Could you check a few things on this model? Use its own coordinates, in mm. Face numbers are marked on the shaded views. A direction names the side the tool comes from. Coordinates: 2 decimals unless noted, no trailing zeros. Write each loop counter-clockwise with the first axis right and the second up, starting at its lowest first coordinate (ties: lowest second). Pieces come first, ordered by that corner, then holes. Notation, with made-up numbers: M -36.75,-17.75 L 11.25,-17.75 A24 cw 11.25,2.25 Z; hole C -17.5,56.25 d8. An arc over 180 degrees is marked long. Write item = value, one per line.
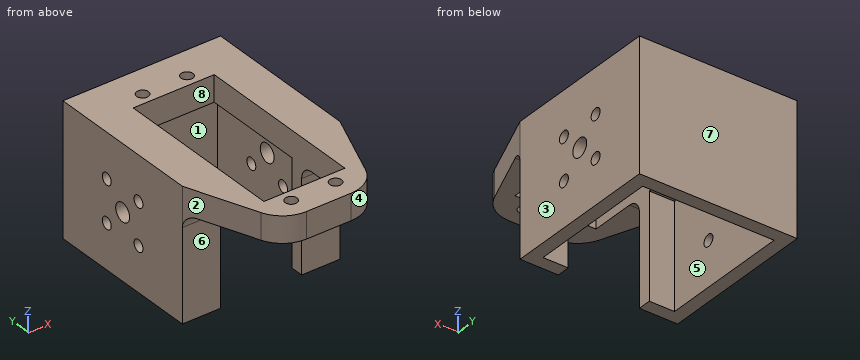
Autodesk Inventor part; units mm, degrees
ref_plane "YZ Plane" through (0, 0, 0) normal (1, 0, 0) x (0, 1, 0)
ref_plane "XZ Plane" through (0, 0, 0) normal (0, 1, 0) x (-1, 0, 0)
ref_plane "XY Plane" through (0, 0, 0) normal (0, 0, 1) x (1, 0, 0)
sketch "Sketch1" plane through (0, 0, 0) normal (0, 0, 1) x (1, 0, 0)
  line L0 (-25.15, 25.15) -> (25.15, 25.15)
  line L1 (25.15, 25.15) -> (25.15, -25.15)
  line L2 (25.15, -25.15) -> (-25.15, -25.15)
  line L3 (-25.15, -25.15) -> (-25.15, 25.15)
  line L4 (-25.15, 25.15) -> (25.15, -25.15) construction
  line L5 (25.15, 25.15) -> (-25.15, -25.15) construction
  line L6 (-30.15, 30.15) -> (30.15, 30.15)
  line L7 (30.15, 30.15) -> (30.15, -30.15)
  line L8 (30.15, -30.15) -> (-30.15, -30.15)
  line L9 (-30.15, -30.15) -> (-30.15, 30.15)
  line L10 (-30.15, 30.15) -> (30.15, -30.15) construction
  line L11 (30.15, 30.15) -> (-30.15, -30.15) construction
  line L12 (0, 25.15) -> (0, 18.5) construction
  line L13 (0, 18.5) -> (8.5, 18.5) construction
  circle A0 centre (8.5, 18.5) radius 2.25
  line L14 (8.5, 18.5) -> (-8.5, 18.5)
  line L15 (-8.5, 18.5) -> (-8.5, -56.5)
  line L16 (-8.5, -56.5) -> (8.5, -56.5)
  line L17 (8.5, -56.5) -> (8.5, 18.5)
  circle A1 centre (8.5, -56.5) radius 2.25
  line L18 (-8.5, 18.5) -> (8.5, -56.5) construction
  line L19 (-15.5, 14) -> (15.5, 14)
  line L20 (15.5, 14) -> (15.5, -52)
  line L21 (15.5, -52) -> (-15.5, -52)
  line L22 (-15.5, -52) -> (-15.5, 14)
  line L23 (-15.5, 14) -> (15.5, -52) construction
  line L24 (15.5, 14) -> (-15.5, -52) construction
  circle A2 centre (-8.5, -56.5) radius 2.25
  circle A3 centre (-8.5, 18.5) radius 2.25
  line L25 (-30.15, -30.15) -> (-20.0032, -56.4398)
  arc A4 (-20.0032, -56.4398) -> (-8.5, -64.3302) centre (-8.5, -52) ccw
  line L26 (0, 0) -> (0, -19) construction
  line L27 (30.15, -30.15) -> (20.0032, -56.4398)
  line L28 (-8.5, -64.3302) -> (8.5, -64.3302)
  arc A5 (8.5, -64.3302) -> (20.0032, -56.4398) centre (8.5, -52) ccw
  point P0 (15.5, -25.15)
  point P1 (15.5, -30.15)
  point P2 (-15.5, -30.15)
  point P3 (-15.5, -25.15)
  dimension "d0" = 50.3
  dimension "d2" = 60.3
  dimension "d4" = 6.65
  dimension "d5" = 8.5
  dimension "d6" = 4.5
  dimension "d7" = 17
  dimension "d8" = 75
  dimension "d10" = 31
  dimension "d11" = 66
extrude "Extrusion1" add sketch "Sketch1" against normal blind 40 contours L3 L2 L22 L8 L9 L6 L7 L20 L1 L0
extrude "Extrusion2" add sketch "Sketch1" along normal blind 10 contours L3 L2 L22 L8 L9 L6 L7 L20 L1 L0 | L0 L1 L2 L20 L19 L17 A0 L14 A3 L15 L22 L3 | L22 L21 L15 A2 L16 A1 L17 L20 L8 L27 A5 L28 A4 L25 | L15 A3 L14 A0 L17 L19 | L21 L17 A1 L16 A2 L15
fillet "Fillet1" radius 5 2 edges at (22.825, -30.15, 0) (-22.825, -30.15, 0)
sketch "Sketch2" plane through (30.15, -30.15, -40) normal (1, 0, 0) x (0, 0, -1)
  line L0 (0, 60.3) -> (0, 0)
  line L1 (-10, 60.3) -> (-40, 60.3)
  line L2 (-40, 60.3) -> (-40, 0)
  line L3 (-40, 0) -> (-10, 0)
  line L4 (-10, 0) -> (-10, 60.3)
  line L5 (-35, 0) -> (0, 0) construction
  circle A0 centre (-25, 30.15) radius 3.5
  line L6 (0.0184, 0) -> (-9.9816, 0) construction
  line L7 (-35, 0) -> (0, 0)
  line L8 (-33, 38.15) -> (-17, 38.15) construction
  line L9 (-17, 38.15) -> (-17, 22.15) construction
  line L10 (-17, 22.15) -> (-33, 22.15) construction
  line L11 (-33, 22.15) -> (-33, 38.15) construction
  line L12 (-33, 38.15) -> (-17, 22.15) construction
  line L13 (-17, 38.15) -> (-33, 22.15) construction
  circle A1 centre (-33, 38.15) radius 2.25
  circle A2 centre (-17, 38.15) radius 2.25
  circle A3 centre (-17, 22.15) radius 2.25
  circle A4 centre (-33, 22.15) radius 2.25
  line L14 (-25, 30.15) -> (-20.3356, 34.8144) construction
  line L15 (-10, 60.3) -> (-40, 0) construction
  line L16 (-25, 30.15) -> (-30.0486, 30.15) construction
  point P0 (-40, 30.15)
  dimension "d20" = 30
  dimension "d21" = 7
  dimension "d24" = 10
  dimension "d25" = 16
  dimension "d27" = 4.5
  dimension "d28" = 60.3
extrude "Extrusion3" cut sketch "Sketch2" against normal blind 65 contours A0 | A1 | A2 | A3 | A4
properties part number "Servo-house" material "PBT Plastic"
Item 1: Imagine slicing it at A-A (y = 8). Write out the boundary of the cut face in (x, z).
Numbers:
outline = M -30.15,-40 L -25.15,-40 L -25.15,-25.25 L -30.15,-25.25 Z; M -30.15,-20.75 L -25.15,-20.75 L -25.15,-9.25 L -30.15,-9.25 Z; M -30.15,-4.75 L -25.15,-4.75 L -25.15,0 L -15.5,0 L -15.5,10 L -30.15,10 Z; M 15.5,0 L 25.15,0 L 25.15,-4.75 L 30.15,-4.75 L 30.15,10 L 15.5,10 Z; M 25.15,-40 L 30.15,-40 L 30.15,-25.25 L 25.15,-25.25 Z; M 25.15,-20.75 L 30.15,-20.75 L 30.15,-9.25 L 25.15,-9.25 Z
Item 2: I'm going to push flat-ended pins straight in: P1, Ø6, axis at y = 8, z = -7, coming from the +X side; P2, Ø1, axis at x = 21, y = -4.5, coming from the -Z side; P3, Ø11.5, axis at x = 20.5, z = -21, coming from the -Y side. Where does each tip first touch, or does it pass through?
Numbers:
P1 = 30.15
P2 = 0
P3 = -30.15
Item 3: Imagine slicing it at C-C (z = -23). Write out the boundary of the cut face in (x, y), and give its area (3 significant figures).
Numbers:
outline = M -30.15,-30.15 L -15.5,-30.15 L -15.5,-25.15 L -25.15,-25.15 L -25.15,-10.25 L -30.15,-10.25 Z; M -30.15,-5.75 L -25.15,-5.75 L -25.15,5.75 L -30.15,5.75 Z; M -30.15,10.25 L -25.15,10.25 L -25.15,25.15 L 25.15,25.15 L 25.15,10.25 L 30.15,10.25 L 30.15,30.15 L -30.15,30.15 Z; M 15.5,-30.15 L 30.15,-30.15 L 30.15,-10.25 L 25.15,-10.25 L 25.15,-25.15 L 15.5,-25.15 Z; M 25.15,-5.75 L 30.15,-5.75 L 30.15,5.75 L 25.15,5.75 Z
area = 861 mm²
Item 4: Imagine slicing it at D-D (y = 18.5). Write out the boundary of the cut face in (x, z), and give its area (3 significant figures).
Numbers:
outline = M -30.15,-40 L -25.15,-40 L -25.15,0 L -10.75,0 L -10.75,10 L -30.15,10 Z; M -6.25,0 L 6.25,0 L 6.25,10 L -6.25,10 Z; M 10.75,0 L 25.15,0 L 25.15,-40 L 30.15,-40 L 30.15,10 L 10.75,10 Z
area = 913 mm²
Item 5: If I drill on line 1 along Y through (x, z) = (26, -23); line 2 along Y through (x, z) = (-18, -29); line 3 along Y through (x, z) = (-8.5, 4), over which ranges is the centre line in solid material (lowest first)?
Numbers:
line_1 = -30.15 to -10.25, -5.75 to 5.75, 10.25 to 30.15
line_2 = -30.15 to -25.15, 25.15 to 30.15
line_3 = -64.33 to -58.75, -54.25 to -52, 14 to 16.25, 20.75 to 30.15
Item 6: Imagine slicing it at B-B (x = -2.5). Write out the boundary of the cut face in (y, z), and give its area (3 significant figures).
Numbers:
outline = M -64.33,0 L -52,0 L -52,10 L -64.33,10 Z; M 14,0 L 25.15,0 L 25.15,-40 L 30.15,-40 L 30.15,10 L 14,10 Z
area = 485 mm²
Item 7: If we mould it in two halves opening along X, with no side actions, what happens to the marked faces 1, 2 and 3? For each: pulls with the +X half, pulls with the -X half, needs draft (parallel to the pull), parting line crosses it, or undercut.
Numbers:
face_1 = undercut
face_2 = pulls with the -X half
face_3 = pulls with the +X half
Item 8: For the marked faces 4, 5, 6, 7 and 8, which set-ups out of +Z, -Z, +X, -X, +Y, -Y let a thin tool reach every point of the face, with its end or its side?
Numbers:
face_4 = +Z, -Z, +X, -Y
face_5 = -Z
face_6 = -Z, +X, -X, -Y
face_7 = +Z, -Z, +X, -X, +Y
face_8 = +Z, -Z
